For this review, take the finished solid that the model builds, in its own axes (mm). Coordinates: 2 decimals unless noted, no trailing zeros. Loops run counter-clockwise (first coordinate to the right, second up) from the corner with the lowest first, then second, coordinate; pieces in that order, holes last. Notation, with made-up numbers: M 61.25,-8.5 L 92.25,-8.5 A14 ccw 92.25,10.5 Z; hole C 75.5,-25 d7. An arc over 180 degrees is marked long. Answer as a JSON object with one key per item and string values. Group by question number.
Item 1: Wall thickness on L1, parallel to Y at x = 11.5, z = 3.7; L2, parallel to Y at x = 184, z = 3.1; L3, parallel to Y at x = 169.9, z = 2.2: over which ranges is each line inside the solid? List them lowest first. Write a range as from..to.
Item 2: Add section A-A (z = 2.2). Count the separate pieces of the cut face and the enclosed holes in it, then the cut area to 3 significant figures.
Item 3: Add section B-B (x = 123). State the section outline as (y, z) points.
Item 4: Insertion check: pin 1 (2.5 mm diameter, centred on y = 31.5, z = 3, fed in from -X); pin 2 (2.5 mm diameter, centred on x = 23.5, z = 2, fed in from +Y); pin 3 (1.4 mm diameter, centred on y = 12.5, z = 1.5, fed in from +X); pin 4 (2 mm diameter, centred on x = 197.2, y = 37.4, fed in from +Z). Each pin has a flat end and moves straight along its axis. Give the tip position at first contact, or say it passes through.
from build123d import *

# Parameters (mm, degrees)
BOSS_EXTRUDE1_DEPTH = 4.7625
SKETCH2_R           = 1.25
SKETCH2_W           = 10
SKETCH2_H           = 5
SKETCH2_W_2         = 7
CUT_EXTRUDE1_DEPTH  = 5.7625


with BuildPart() as part:
    # Sketch1 → Boss-Extrude1 (new body)
    with BuildSketch(Plane.XY):
        Polygon((174.6, 40.2), (150.776470588, 24), (0, 24), (0, 0), (190, 0), (200, 25), (200, 40.2), align=None)
    extrude(amount=BOSS_EXTRUDE1_DEPTH)

    # Sketch2 → Cut-Extrude1 (cut, through all)
    with BuildSketch(Plane.XY.offset(4.7625)):
        with Locations((169.9, 31.1)):
            Circle(SKETCH2_R)
        with Locations((197.2, 37.4)):
            Circle(SKETCH2_R)
        with Locations((169.9, 9.1)):
            Circle(SKETCH2_R)
        with Locations((23.5, 21.2)):
            Circle(SKETCH2_R)
        with Locations((11.5, 21.2)):
            Circle(SKETCH2_R)
        with Locations((11.5, 2.8)):
            Circle(SKETCH2_R)
        with Locations((23.5, 2.8)):
            Circle(SKETCH2_R)
        with Locations((180.1, 31.7)):
            Rectangle(SKETCH2_W, SKETCH2_H)
        with Locations((180.1, 8.5)):
            Rectangle(SKETCH2_W, SKETCH2_H)
        with Locations((11, 12)):
            Rectangle(SKETCH2_W_2, SKETCH2_H)
        with Locations((24, 12)):
            Rectangle(SKETCH2_W_2, SKETCH2_H)
    extrude(amount=-CUT_EXTRUDE1_DEPTH, mode=Mode.SUBTRACT)


solid = part.part
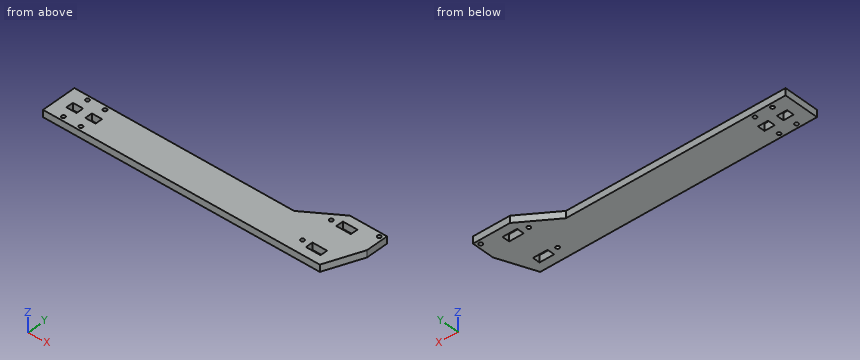
From the geometry:
{
 "1": {"L1": "y = 0..1.55, 4.05..9.5, 14.5..19.95, 22.45..24", "L2": "y = 0..6, 11..29.2, 34.2..40.2", "L3": "y = 0..7.85, 10.35..29.85, 32.35..37"},
 "2": {"separate pieces": "1", "enclosed holes": "11", "area": "5,080 mm²"},
 "3": {"outline": "M 0,0 L 24,0 L 24,4.76 L 0,4.76 Z"},
 "4": {"pin 1": "stops at x = 159.97", "pin 2": "stops at y = 24", "pin 3": "stops at x = 195.28", "pin 4": "passes through"}
}
